```python
from build123d import *

# Parameters (mm, degrees)
SKETCH6_R           = 23
BOSS_EXTRUDE3_DEPTH = 25
SKETCH7_R           = 1.5
CUT_EXTRUDE2_DEPTH  = 5
SKETCH8_R           = 1.25
CUT_EXTRUDE3_DEPTH  = 5
SKETCH9_R           = 4
BOSS_EXTRUDE4_DEPTH = 2
SKETCH10_R          = 2
BOSS_EXTRUDE5_DEPTH = 3
FILLET1_R           = 5
FILLET2_R           = 2
SKETCH11_W          = 58.747444177
SKETCH11_H          = 21.595633685
CUT_EXTRUDE4_DEPTH  = 50
SKETCH12_R          = 20
CUT_EXTRUDE5_DEPTH  = 5


with BuildPart() as part:
    # Sketch6 → Boss-Extrude3 (new body)
    with BuildSketch(Plane(origin=(0, 0, 0), x_dir=(1, 0, 0), z_dir=(0, 1, 0))):
        with Locations(Location((0, 0, 0), (0, 0, 270))):
            Circle(SKETCH6_R)
    extrude(amount=BOSS_EXTRUDE3_DEPTH)

    # Sketch7 → Cut-Extrude2 (cut)
    with BuildSketch(Plane(origin=(0, 0, 0), x_dir=(1, 0, 0), z_dir=(0, 1, 0))):
        with Locations(Location((-6, 0, 0), (0, 0, 270))):
            Circle(SKETCH7_R)
        with Locations(Location((0, 6, 0), (0, 0, 270))):
            Circle(SKETCH7_R)
        with Locations(Location((6, 0, 0), (0, 0, 270))):
            Circle(SKETCH7_R)
        with Locations(Location((0, -6, 0), (0, 0, 270))):
            Circle(SKETCH7_R)
    extrude(amount=CUT_EXTRUDE2_DEPTH, mode=Mode.SUBTRACT)

    # Sketch8 → Cut-Extrude3 (cut)
    with BuildSketch(Plane(origin=(0, 25, 0), x_dir=(1, 0, 0), z_dir=(0, 1, 0))):
        with Locations(Location((-13.856406461, -8, 0), (0, 0, 270))):
            Circle(SKETCH8_R)
        with Locations(Location((0, 16, 0), (0, 0, 270))):
            Circle(SKETCH8_R)
        with Locations(Location((13.856406461, -8, 0), (0, 0, 270))):
            Circle(SKETCH8_R)
    extrude(amount=-CUT_EXTRUDE3_DEPTH, mode=Mode.SUBTRACT)

    # Sketch9 → Boss-Extrude4 (add)
    with BuildSketch(Plane(origin=(0, 25, 0), x_dir=(1, 0, 0), z_dir=(0, 1, 0))):
        with Locations(Location((0, 0, 0), (0, 0, 270))):
            Circle(SKETCH9_R)
    extrude(amount=BOSS_EXTRUDE4_DEPTH)

    # Sketch10 → Boss-Extrude5 (add)
    with BuildSketch(Plane.XZ):
        with Locations(Location((0, 0, 0), (0, 0, 90))):
            Circle(SKETCH10_R)
    extrude(amount=BOSS_EXTRUDE5_DEPTH)

    # Fillet1
    fillet1_edges = [part.edges().sort_by_distance(p)[0] for p in [
        (0, 0, -23),
    ]]
    fillet(fillet1_edges, radius=FILLET1_R)

    # Fillet2
    fillet2_edges = [part.edges().sort_by_distance(p)[0] for p in [
        (0, 25, -23),
    ]]
    fillet(fillet2_edges, radius=FILLET2_R)

    # Sketch11 → Cut-Extrude4 (cut, symmetric)
    with BuildSketch(Plane(origin=(0, 0, 0), x_dir=(0, 0, -1), z_dir=(1, 0, 0))):
        with Locations((0.983000007, 20.797816843)):
            Rectangle(SKETCH11_W, SKETCH11_H)
    extrude(amount=CUT_EXTRUDE4_DEPTH, both=True, mode=Mode.SUBTRACT)

    # Sketch12 → Cut-Extrude5 (cut)
    with BuildSketch(Plane(origin=(0, 10, 0), x_dir=(1, 0, 0), z_dir=(0, 1, 0))):
        with Locations(Location((0, 0, 0), (0, 0, 270))):
            Circle(SKETCH12_R)
    extrude(amount=-CUT_EXTRUDE5_DEPTH, mode=Mode.SUBTRACT)


solid = part.part
```
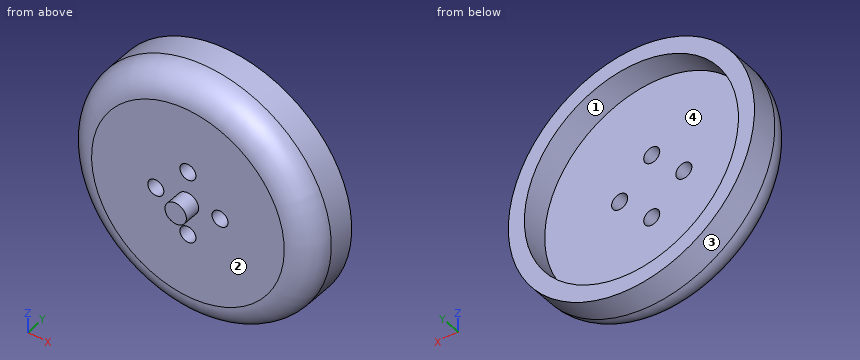
The model under review builds one solid part; all positions refer to its coordinate system, in mm. Face numbers are marked on the shaded views. Round coordinates to 2 decimals unless told otherwise and drop trailing zeros. Loops run counter-clockwise (first coordinate to the right, second up) from the corner with the lowest first, then second, coordinate; pieces in that order, holes last. Notation, with made-up numbers: (76, -20.75) - (105, -20.75) arc R30 ccw to (105, 1.25) - close; hole circle Ø3 at (51, 58). An arc over 180 degrees is marked (long way). Use a Markdown table: item, result. Add a question column.
Q1. Add section D-D (y = 3). State the section outline as (x, z) points, plus the area to 3 significant figures.
Q2. The part is to be moulded in two halves that separate along Z. For the marked faces 1, 2, 3 and 4, say which applies: pulls with the +Z half, pulls with the -Z half, needs draft (parallel to the pull), parting line crosses it, or undercut.
Q3. Add section A-A (z = 0). State the section outline as (x, y) points.
Q4. For probe 1 along X at (y, z) = (8.6, 0); probe 2 along X at (y, z) = (2.35, 0); probe 3 along Y at (x, z) = (-8, 12.5), list the stretches that pass through material, from the lowest coordinate up.
Q5. Add section B-B (x = 0). State the section outline as (y, z) points.
Q6. Add section C-C (y = 9.25). State the section outline as (x, z) points.
Q7. Insertion check: pin 1 Ø4 at (x, z) = (-6, 0) entering from +Y; pin 2 Ø5 at (y, z) = (2, 1.5) entering from +X; pin 3 Ø1 at (y, z) = (1.5, 4.5) entering from -X. Each pin has a flat end and moves straight along its axis. Give the tip position at first contact, or say it passes through.
Worked answers:
| question | item | result |
|---|---|---|
| 1 | outline | circle Ø45.17 at (0, 0); hole circle Ø3 at (-6, 0); hole circle Ø3 at (0, -6); hole circle Ø3 at (0, 6); hole circle Ø3 at (6, 0) |
| 1 | area | 1,570 mm² |
| 2 | face 1 | undercut |
| 2 | face 2 | needs draft |
| 2 | face 3 | parting line crosses it |
| 2 | face 4 | undercut |
| 3 | outline | (-23, 5) arc R5 ccw to (-18, 0) - (-7.5, 0) - (-7.5, 5) - (-20, 5) - (-20, 10) - (-23, 10) - close; (-4.5, 0) - (-2, 0) - (-2, -3) - (2, -3) - (2, 0) - (4.5, 0) - (4.5, 5) - (-4.5, 5) - close; (7.5, 0) - (18, 0) arc R5 ccw to (23, 5) - (23, 10) - (20, 10) - (20, 5) - (7.5, 5) - close |
| 4 | probe 1 | -23 to -20, 20 to 23 |
| 4 | probe 2 | -22.24 to -7.5, -4.5 to 4.5, 7.5 to 22.24 |
| 4 | probe 3 | 0 to 5 |
| 5 | outline | (-3, -2) - (0, -2) - (0, -4.5) - (5, -4.5) - (5, 4.5) - (0, 4.5) - (0, 2) - (-3, 2) - close; (0, -18) arc R5 ccw to (5, -23) - (10, -23) - (10, -20) - (5, -20) - (5, -7.5) - (0, -7.5) - close; (0, 7.5) - (5, 7.5) - (5, 20) - (10, 20) - (10, 23) - (5, 23) arc R5 ccw to (0, 18) - close |
| 6 | outline | circle Ø46 at (0, 0); hole circle Ø40 at (0, 0) |
| 7 | pin 1 | y = 5 |
| 7 | pin 2 | x = 22.95 |
| 7 | pin 3 | x = -21.55 |
